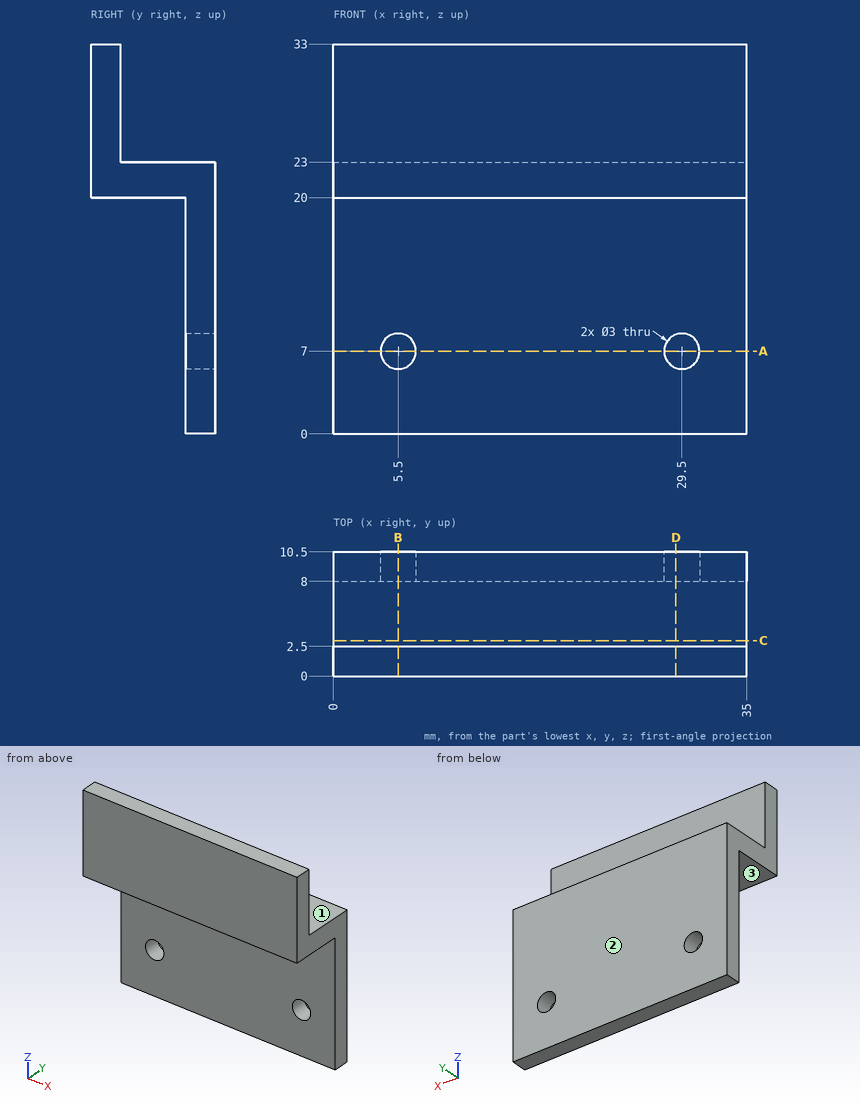
The drawing under review shows one solid part. Ordinate dimensions are in mm from its lowest x, y, z. A direction names the side the tool comes from. Coordinates: 2 decimals unless noted, no trailing zeros. Write each loop counter-clockwise with the first axis right and the second up, starting at its lowest first coordinate (ties: lowest second). Pieces come first, ordered by that corner, then holes.
1) Add section C-C (y = 3). Write out the cut boundary in (x, z), plus the area to 3 significant figures.
2) Add section B-B (x = 5.5). Write out the cut boundary in (y, z).
3) Add section D-D (x = 29). Write out the cut boundary in (y, z).
4) Machinability: for the marked faces 1, 2 and 3, which of the approach directions +Z, -Z, +X, -X, +Y, -Y give a long, thin tool a straight path to every point of the face, cutting with its end or side? Answer none if there is none.
5) Insertion check: pin 1 (4 mm diameter, centred on x = 20.5, y = 2.5, fed in from -Z); pin 2 (4 mm diameter, centred on x = 5.5, z = 7, fed in from -Y); pin 3 (4 mm diameter, centred on x = 18, y = 7, fed in from +Z). Each pin has a flat end and moves straight along its axis. Give the tip position at first contact, or say it passes through.
6) To check wall thickness, follow L1, parallel to Z at x = 5.5, y = 9.3; L2, parallel to Z at x = 33, y = 10; L3, parallel to Y at x = 33, z = 11. State the ranges of each line that lie inside material, in increasing order.
7) Add section A-A (z = 7). Write out the cut boundary in (x, y).
Check result:
1. outline: (0, 20) - (35, 20) - (35, 23) - (0, 23) - close
1. area: 105 mm2
2. outline: (0, 20) - (8, 20) - (8, 8.5) - (10.5, 8.5) - (10.5, 23) - (2.5, 23) - (2.5, 33) - (0, 33) - close; (8, 0) - (10.5, 0) - (10.5, 5.5) - (8, 5.5) - close
3. outline: (0, 20) - (8, 20) - (8, 8.41) - (10.5, 8.41) - (10.5, 23) - (2.5, 23) - (2.5, 33) - (0, 33) - close; (8, 0) - (10.5, 0) - (10.5, 5.59) - (8, 5.59) - close
4. face 1: +Z, +X, -X, +Y
4. face 2: +Z, -Z, +X, -X, +Y
4. face 3: -Z, +X, -X, -Y
5. pin 1: stops at z = 20
5. pin 2: stops at y = 8
5. pin 3: stops at z = 23
6. L1: z = 0 to 5.5, 8.5 to 23
6. L2: z = 0 to 23
6. L3: y = 8 to 10.5
7. outline: (0, 8) - (4, 8) - (4, 10.5) - (0, 10.5) - close; (7, 8) - (28, 8) - (28, 10.5) - (7, 10.5) - close; (31, 8) - (35, 8) - (35, 10.5) - (31, 10.5) - close
